Design review of the part built by this model. Coordinates are the model's own, in mm. A direction names the side the tool comes from. Round coordinates to 2 decimals unless told otherwise and drop trailing zeros. Order: outer loops, then holes, each group sorted by start corner. A loop starts at its lowest first (then second) coordinate and runs counter-clockwise, first axis right, second up. Notation, with made-up numbers: (10.25, -33.75) - (19.25, -33.75) arc R4 ccw to (19.25, -27.75) - close; hole circle Ø10 at (-27.75, 57.25). An arc over 180 degrees is marked (long way). Write item = value, one per line.
from build123d import *

# Parameters (mm, degrees)
SKETCH1_R           = 11.495405
BOSS_EXTRUDE2_DEPTH = 4.7625
BOSS_EXTRUDE3_DEPTH = 3.175
FILLET1_R           = 1.5875


with BuildPart() as part:
    # Sketch1 → Boss-Extrude2 (new, symmetric)
    with BuildSketch(Plane.XY):
        with BuildLine():
            ThreePointArc((14.672983865, 0.491098707), (-4.158599684, 14.079903484), (-12.585193267, -7.559797873))
            ThreePointArc((-12.585193267, -7.559797873), (4.158599684, -14.079903484), (14.672983865, 0.491098707))
        make_face()
        with Locations(Location((0, 0, 0), (0, 0, 180))):
            Circle(SKETCH1_R, mode=Mode.SUBTRACT)
    extrude(amount=BOSS_EXTRUDE2_DEPTH, both=True)

    # Sketch1_4 → Boss-Extrude3 (add, symmetric)
    with BuildSketch(Plane.XY):
        with BuildLine():
            ThreePointArc((-12.585193267, -7.559797873), (-10.89585042, -11.492870345), (-10.31875, -15.734319794))
            Line((-10.31875, -15.734319794), (-10.31875, -56.374319794))
            Line((-10.31875, -56.374319794), (8.54075, -56.374319794))
            Line((8.54075, -56.374319794), (8.54075, -100.824319794))
            Line((8.54075, -100.824319794), (47.609422672, -89.285109315))
            Line((47.609422672, -89.285109315), (23.458960581, -51.968120144))
            Line((23.458960581, -51.968120144), (39.292025986, -41.721424085))
            Line((39.292025986, -41.721424085), (17.211603503, -7.603033986))
            ThreePointArc((17.211603503, -7.603033986), (15.391641433, -3.728672569), (14.672983865, 0.491098707))
            ThreePointArc((14.672983865, 0.491098707), (4.158599684, -14.079903484), (-12.585193267, -7.559797873))
        make_face()
        with BuildLine():
            ThreePointArc((5.55625, -46.055569794), (0, -51.611819794), (-5.55625, -46.055569794))
            Line((-5.55625, -46.055569794), (-5.55625, -34.943069794))
            ThreePointArc((-5.55625, -34.943069794), (0, -29.386819794), (5.55625, -34.943069794))
            Line((5.55625, -34.943069794), (5.55625, -46.055569794))
        make_face(mode=Mode.SUBTRACT)
        with BuildLine():
            ThreePointArc((29.687419875, -35.646101109), (28.04160399, -43.329532516), (20.358172583, -41.683716631))
            Line((20.358172583, -41.683716631), (14.32055706, -32.354469339))
            ThreePointArc((14.32055706, -32.354469339), (15.966372945, -24.671037931), (23.649804353, -26.316853816))
            Line((23.649804353, -26.316853816), (29.687419875, -35.646101109))
        make_face(mode=Mode.SUBTRACT)
    extrude(amount=BOSS_EXTRUDE3_DEPTH, both=True)

    # Fillet1
    fillet1_edges = [part.edges().sort_by_distance(p)[0] for p in [
        (47.609422672, -89.285109315, 0),
        (23.458960581, -51.968120144, 0),
        (39.292025986, -41.721424085, 0),
        (-10.31875, -56.374319794, 0),
        (8.54075, -56.374319794, 0),
        (8.54075, -100.824319794, 0),
    ]]
    fillet(fillet1_edges, radius=FILLET1_R)


solid = part.part
Item 1: Take a section at B-B, the plane y = -48.5. State the section outline as (x, z) points (3 decimals).
Data:
outline = (-10.319, -3.175) - (-4.99, -3.175) - (-4.99, 3.175) - (-10.319, 3.175) - close; (4.99, -3.175) - (28.818, -3.175) - (28.818, 3.175) - (4.99, 3.175) - close
Item 2: For faces 1 (the face through (31.283, -46.904, 0.044)), 2 (the face through (-5.556, -41, 0)), 3 (the face through (8.541, -78, 0)), 4 (the face through (27.97, -24.23, 0.04)), list the 3-axis set-ups (+Z, -Z, +X, -X, +Y, -Y) from which the entire face can be reached by the end or side of a thin tool; tool diameter is ignored.
Data:
face_1 = +Z, -Z, +X
face_2 = +Z, -Z
face_3 = +Z, -Z, -X, -Y
face_4 = +Z, -Z, +X, +Y
Item 3: For line 1 along Y through (x, z) = (0, 1.25); line 2 along Y through (x, z) = (-1.5, -0.25); line 3 along Y through (x, z) = (0, 3.6), list the stretches that pass through material, from the lowest coordinate up. Write a range as [from, to].
Data:
line_1 = [-56.37, -51.61], [-29.39, -11.5], [11.5, 14.68]
line_2 = [-56.37, -51.41], [-29.59, -11.4], [11.4, 14.6]
line_3 = [-14.68, -11.5], [11.5, 14.68]
Item 4: Insertion check: P1, Ø18, axis at x = 28, y = -36.5, coming from the +Z side (3 decimals); P2, Ø3, axis at y = -30.5, z = 3, coming from the -X side; P3, Ø5, axis at x = 13.5, z = -1.5, coming from the -Y side. Each pin has a flat end and moves straight along its axis. Give the tip position at first contact, or say it passes through.
Data:
P1 = 3.175
P2 = -10.32
P3 = -100.1
Item 5: Take a section at D-D, the plane y = 5. State the section outline as (x, z) points, and give its area (3 significant figures).
Data:
outline = (-13.8, -4.76) - (-10.35, -4.76) - (-10.35, 4.76) - (-13.8, 4.76) - close; (10.35, -4.76) - (13.8, -4.76) - (13.8, 4.76) - (10.35, 4.76) - close
area = 65.8 mm2
Item 6: The part is to be moulded in two halves that separate along Y. For faces 5 (the face through (-0.12, -29.39, 0.04)), 6 (the face through (17, -60, 3.175)), 7 (the face through (46.604, -88.935, 0.044)), say which applies: +Y half, -Y half, draft (parallel to the pull), parting line (faces both ways), or undercut.
Data:
face_5 = undercut
face_6 = draft
face_7 = parting line
Item 7: Take a section at A-A, the plane x = 0. State the section outline as (y, z) points (1 decimal).
Data:
outline = (-56.4, -3.2) - (-51.6, -3.2) - (-51.6, 3.2) - (-56.4, 3.2) - close; (-29.4, -3.2) - (-14.7, -3.2) - (-14.7, -4.8) - (-11.5, -4.8) - (-11.5, 4.8) - (-14.7, 4.8) - (-14.7, 3.2) - (-29.4, 3.2) - close; (11.5, -4.8) - (14.7, -4.8) - (14.7, 4.8) - (11.5, 4.8) - close
Item 8: Take a section at C-C, the plane z = -1.25. Count the separate pieces of the cut face and the enclosed holes in it, and give its area (3 significant figures).
Data:
separate_pieces = 1
enclosed_holes = 3
area = 2,770 mm2
